```python
from build123d import *

# Parameters (mm, degrees)
SKETCH_W     = 12.8
SKETCH_H     = 6.2
PAD_DEPTH    = 2.9
SKETCH001_W  = 0.8
SKETCH001_H  = 0.4
PAD001_DEPTH = 2.8
PAD002_DEPTH = 1.825
SKETCH003_R  = 1
POCKET_DEPTH = 5.801


with BuildPart() as part:
    # Sketch → Pad (new body, symmetric)
    with BuildSketch(Plane.XY):
        Rectangle(SKETCH_W, SKETCH_H)
    extrude(amount=PAD_DEPTH, both=True)

    # Sketch001 (on Face3 of Pad) → Pad001 (join)
    with BuildSketch(Plane.XZ.offset(3.1)):
        with Locations((-5.1, 0)):
            Rectangle(SKETCH001_W, SKETCH001_H)
        Rectangle(SKETCH001_W, SKETCH001_H)
        with Locations((5.1, 0)):
            Rectangle(SKETCH001_W, SKETCH001_H)
    extrude(amount=PAD001_DEPTH)

    # Sketch002 → Pad002 (join, symmetric)
    with BuildSketch(Plane.XY):
        Polygon((4.230478, 3.1), (-6.4, 6.969178), (-6.263192, 7.345055), (5.4, 3.1), align=None)
    extrude(amount=PAD002_DEPTH, both=True)

    # Sketch003 (on Face4 of Pad002) → Pocket (cut, through all)
    with BuildSketch(Plane.XY.offset(2.9)):
        with Locations((-3.2, -1.57)):
            Circle(SKETCH003_R)
        with Locations((3.2, -1.57)):
            Circle(SKETCH003_R)
    extrude(amount=-POCKET_DEPTH, mode=Mode.SUBTRACT)


solid = part.part
```
Here's how the part is built. I have some questions about the finished solid (model axes, mm). A direction names the side the tool comes from. Give positions to 0.01 mm unless a question says otherwise; leave off trailing zeros. Loops run counter-clockwise (first coordinate to the right, second up) from the corner with the lowest first, then second, coordinate; pieces in that order, holes last. Notation, with made-up numbers: M 49,-18 L 58,-18 A26 ccw 58,9 Z; hole C 89,37.25 d4. An arc over 180 degrees is marked long. Use one line per item in the form item = value. Start each with the question number.
Q1. Thinking about a two-plate mould opening in Y: for faces 1 (the flat face through (0, 0, 2.9)), 2 (the cylindrical face through (2.2, -1.53, 0.04)), 3 (the flat face through (-0.51, 5.25, 0.03)), which applies, +Y half, -Y half, draft (parallel to the pull), parting line (faces both ways), or undercut?
Q2. Will these pins go through, and if not, where does the flat tip stop? pin 1 Ø2 at (x, y) = (-1.5, 6) entering from +Z (3 decimals); pin 2 Ø1.7 at (x, z) = (1.5, 1) entering from -Y.
Q3. I need wall thicknesses on line 1 along Y through (x, z) = (-3, 0.95); line 2 along Y through (x, z) = (3.2, -1.1); line 3 along Y through (x, z) = (-1.75, -2.35). Which ranges of each line are inside material? Lowest first, please.
Q4. If we section it at C-C (z = -2.4): Write out the boundary of the cut face in (x, y).
Q5. If we section it at A-A (y = -3.75): Write out the boundary of the cut face in (x, z).
Q6. If we section it at D-D (x = -3.2): Write out the boundary of the cut face in (y, z) (3 decimals).
Q7. Which directions (+Z, -Z, +X, -X, +Y, -Y) give clear straight access to the entire face, cutting with the end or side of a thin tool? Please do faces 4 (the flat face through (-5, -4, 0.2)), 5 (the flat face through (-5, -4, -0.2)), 6 (the flat face through (-1.35, 5.39, -1.825)), 7 (the flat face through (-1.35, 5.39, 1.825)).
Q8. If we section it at B-B (x = -1): Write out the boundary of the cut face in (y, z) (3 decimals), then the cut area to 3 significant figures.
Taken from the geometry:
q1.face_1 = draft
q1.face_2 = undercut
q1.face_3 = +Y half
q2.pin_1 = 1.825
q2.pin_2 = -3.1
q3.line_1 = -3.1 to -2.55, -0.59 to 3.1, 5.73 to 6.16
q3.line_2 = -3.1 to -2.57, -0.57 to 3.1, 3.48 to 3.9
q3.line_3 = -3.1 to 3.1
q4.outline = M -6.4,-3.1 L 6.4,-3.1 L 6.4,3.1 L -6.4,3.1 Z; hole C -3.2,-1.57 d2; hole C 3.2,-1.57 d2
q5.outline = M -5.5,-0.2 L -4.7,-0.2 L -4.7,0.2 L -5.5,0.2 Z; M -0.4,-0.2 L 0.4,-0.2 L 0.4,0.2 L -0.4,0.2 Z; M 4.7,-0.2 L 5.5,-0.2 L 5.5,0.2 L 4.7,0.2 Z
q6.outline = M -3.1,-2.9 L -2.57,-2.9 L -2.57,2.9 L -3.1,2.9 Z; M -0.57,-2.9 L 3.1,-2.9 L 3.1,2.9 L -0.57,2.9 Z; M 5.804,-1.825 L 6.23,-1.825 L 6.23,1.825 L 5.804,1.825 Z
q7.face_4 = +Z, +X, -X, -Y
q7.face_5 = -Z, +X, -X, -Y
q7.face_6 = -Z, +X, -X, +Y
q7.face_7 = +Z, +X, -X, +Y
q8.outline = M -3.1,-2.9 L 3.1,-2.9 L 3.1,2.9 L -3.1,2.9 Z; M 5.004,-1.825 L 5.429,-1.825 L 5.429,1.825 L 5.004,1.825 Z
q8.area = 37.5 mm^2
